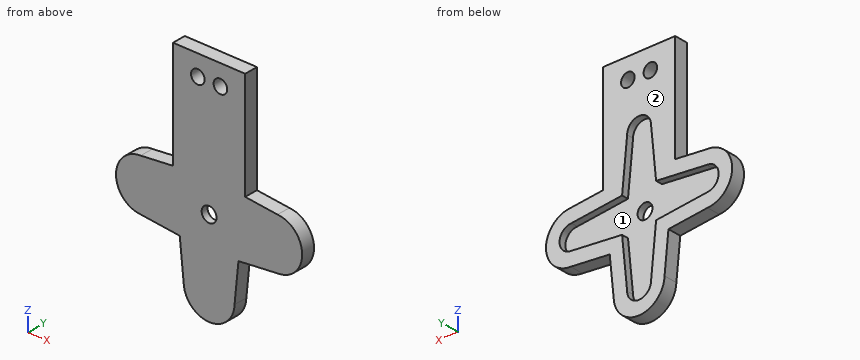
```python
from build123d import *
from build123d.topology import SkipClean

# Parameters (mm, degrees)
SKETCH1_R               = 21
BOSS_EXTRUDE1_DEPTH     = 1.5
SKETCH2_R               = 2.65
CUT_EXTRUDE1_DEPTH      = 1.5
SKETCH5_W               = 16
SKETCH5_H               = 30
BOSS_EXTRUDE2_DEPTH     = 1.5
CIRPATTERN1_DEPTH       = 1.5
CUT_EXTRUDE4_REACH      = 38.65
SKETCH4_R               = 1.65
CUT_EXTRUDE5_REACH      = 38.742
SKETCH6_R               = 1.5
CUT_EXTRUDE6_DEPTH      = 37.650375169
CUT_EXTRUDE6_DEPTH_BACK = 37.650375169


# Read off the part's stored shape, not the designer's step: CirPattern1
with BuildPart() as part:
    # Sketch1 → Boss-Extrude1 (new, symmetric)
    with BuildSketch(Plane(origin=(0, 0, 0), x_dir=(1, 0, 0), z_dir=(0, 1, 0))):
        with Locations(Location((0, 0, 0), (0, 0, 270))):
            Circle(SKETCH1_R)
    extrude(amount=BOSS_EXTRUDE1_DEPTH, both=True)

    # Sketch2 → Cut-Extrude1 (cut)
    with BuildSketch(Plane(origin=(0, 1.5, 0), x_dir=(1, 0, 0), z_dir=(0, 1, 0))):
        with Locations((0, -15)):
            Circle(SKETCH2_R)
        with BuildLine():
            ThreePointArc((-2.65, -15), (0, -12.35), (2.65, -15))
            Line((2.65, -15), (4.067821782, -0.821782178))
            ThreePointArc((4.067821782, -0.821782178), (0, -4.15), (-4.067821782, -0.821782178))
            Line((-4.067821782, -0.821782178), (-2.65, -15))
        make_face()
        with BuildLine():
            ThreePointArc((-4.067821782, -0.821782178), (0, -4.15), (4.067821782, -0.821782178))
            Line((4.067821782, -0.821782178), (4.15, 0))
            ThreePointArc((4.15, 0), (0, 4.15), (-4.15, 0))
            Line((-4.15, 0), (-4.067821782, -0.821782178))
        make_face()
    cut_extrude1 = extrude(amount=-CUT_EXTRUDE1_DEPTH, mode=Mode.SUBTRACT)

    # Sketch5 → Boss-Extrude2 (add, symmetric)
    with BuildSketch(Plane(origin=(0, 0, 0), x_dir=(1, 0, 0), z_dir=(0, 1, 0))):
        with Locations((0, -15)):
            Rectangle(SKETCH5_W, SKETCH5_H)
    extrude(amount=BOSS_EXTRUDE2_DEPTH, both=True)

    # Mirror1: Cut-Extrude1 across plane
    with SkipClean():  # the faces are left unmerged after this step: merging them gives an invalid solid
        add(cut_extrude1.mirror(Plane.XY), mode=Mode.SUBTRACT)

    # CirPattern1 outline → CirPattern1 (cut)
    with BuildSketch(Plane(origin=(0, 0, 0), x_dir=(1, 0, 0), z_dir=(0, 1, 0))):
        with BuildLine():
            Line((3.772727273, -3.772727273), (15, -2.65))
            ThreePointArc((15, -2.65), (17.65, 0), (15, 2.65))
            Line((15, 2.65), (3.772727273, 3.772727273))
            Line((3.772727273, 3.772727273), (4.067821782, 0.821782178))
            ThreePointArc((4.067821782, 0.821782178), (0, -4.15), (-4.067821782, 0.821782178))
            Line((-4.067821782, 0.821782178), (-3.772727273, 3.772727273))
            Line((-3.772727273, 3.772727273), (-15, 2.65))
            ThreePointArc((-15, 2.65), (-17.65, 0), (-15, -2.65))
            Line((-15, -2.65), (-3.772727273, -3.772727273))
            Line((-3.772727273, -3.772727273), (-2.65, -15))
            ThreePointArc((-2.65, -15), (0, -17.65), (2.65, -15))
            Line((2.65, -15), (3.772727273, -3.772727273))
        make_face()
    extrude(amount=CIRPATTERN1_DEPTH, mode=Mode.SUBTRACT)

    # Sketch4 → Cut-Extrude4 (cut, up to next)
    with BuildSketch(Plane(origin=(0, 0, 0), x_dir=(1, 0, 0), z_dir=(0, 1, 0)), mode=Mode.PRIVATE) as cut_extrude4_sk1:
        with Locations(Location((0, 0, 0), (0, 0, 270))):
            Circle(SKETCH4_R)
    cut_extrude4_tool1 = extrude(cut_extrude4_sk1.sketch, amount=-CUT_EXTRUDE4_REACH, mode=Mode.PRIVATE) & part.part
    add(cut_extrude4_tool1.solids().sort_by_distance((0, 0, 0))[0], mode=Mode.SUBTRACT)

    # Sketch6 → Cut-Extrude5 (cut, up to next)
    with BuildSketch(Plane(origin=(0, 1.5, 0), x_dir=(1, 0, 0), z_dir=(0, 1, 0)), mode=Mode.PRIVATE) as cut_extrude5_sk1:
        with Locations(Location((2.5, -25.5, 0), (0, 0, 270))):
            Circle(SKETCH6_R)
    cut_extrude5_tool1 = extrude(cut_extrude5_sk1.sketch, amount=-CUT_EXTRUDE5_REACH, mode=Mode.PRIVATE) & part.part
    # Sketch6 → Cut-Extrude5 (cut, up to next)
    with BuildSketch(Plane(origin=(0, 1.5, 0), x_dir=(1, 0, 0), z_dir=(0, 1, 0)), mode=Mode.PRIVATE) as cut_extrude5_sk2:
        with Locations(Location((-2.5, -25.5, 0), (0, 0, 270))):
            Circle(SKETCH6_R)
    cut_extrude5_tool2 = extrude(cut_extrude5_sk2.sketch, amount=-CUT_EXTRUDE5_REACH, mode=Mode.PRIVATE) & part.part
    add(cut_extrude5_tool1.solids().sort_by_distance((2.5, 1.5, 25.5))[0], mode=Mode.SUBTRACT)
    add(cut_extrude5_tool2.solids().sort_by_distance((-2.5, 1.5, 25.5))[0], mode=Mode.SUBTRACT)

    # Sketch7 → Cut-Extrude6 (cut, two sides: drawn at the far end of the back side and taken through both)
    with BuildSketch(Plane(origin=(0, 0, 0), x_dir=(1, 0, 0), z_dir=(0, 1, 0)).offset(-CUT_EXTRUDE6_DEPTH_BACK)):
        with BuildLine():
            ThreePointArc((8, -19.416487839), (0, 21), (-8, -19.416487839))
            Line((-8, -19.416487839), (-8, -6.364962686))
            Line((-8, -6.364962686), (-15.177522436, -5.647210443))
            ThreePointArc((-15.177522436, -5.647210443), (-20.65, 0), (-15.177522436, 5.647210443))
            Line((-15.177522436, 5.647210443), (-6.513602442, 6.513602442))
            Line((-6.513602442, 6.513602442), (-5.647210443, 15.177522436))
            ThreePointArc((-5.647210443, 15.177522436), (0, 20.65), (5.647210443, 15.177522436))
            Line((5.647210443, 15.177522436), (6.513602442, 6.513602442))
            Line((6.513602442, 6.513602442), (15.177522436, 5.647210443))
            ThreePointArc((15.177522436, 5.647210443), (20.65, 0), (15.177522436, -5.647210443))
            Line((15.177522436, -5.647210443), (8, -6.364962686))
            Line((8, -6.364962686), (8, -19.416487839))
        make_face()
    extrude(amount=CUT_EXTRUDE6_DEPTH + CUT_EXTRUDE6_DEPTH_BACK, mode=Mode.SUBTRACT)


solid = part.part
```
Design review of the part built by this model. Coordinates are the model's own, in mm. Face numbers are marked on the shaded views. Give positions to 0.01 mm unless a question says otherwise; leave off trailing zeros. Loops run counter-clockwise (first coordinate to the right, second up) from the corner with the lowest first, then second, coordinate; pieces in that order, holes last. Notation, with made-up numbers: (33, 62) -> (86, 62) arc R27 ccw to (86, 85) -> close; hole circle Ø4 at (-3.5, 55). An arc over 180 degrees is marked (long way). Write each question's results on one line, items separated by ' | '.
Q1. Wall thickness on L1, parallel to X at y = -0.7, z = 25.5; L2, parallel to Z at x = 2, y = 0.35; L3, parallel to X at y = -1.05, z = 0: over which ranges is each line inside the solid? List them lowest first.
Reply:
L1: x = -8 to -4, -1 to 1, 4 to 8 | L2: z = -20.28 to -16.74, 16.74 to 24.09, 26.91 to 30 | L3: x = -20.65 to -1.65, 1.65 to 20.65
Q2. Take a section at B-B, the plane z = 25.5. Write out the cut boundary in (x, y).
Reply:
outline: (-8, -1.5) -> (-4, -1.5) -> (-4, 1.5) -> (-8, 1.5) -> close; (-1, -1.5) -> (1, -1.5) -> (1, 1.5) -> (-1, 1.5) -> close; (4, -1.5) -> (8, -1.5) -> (8, 1.5) -> (4, 1.5) -> close
Q3. For pin 1 Ø0.9 at (y, z) = (0.5, 12.5) entering from +X; pin 2 Ø1.8 at (x, z) = (-2.5, 25.5) entering from -Y, all flat-tipped, find the tip position at first contact; note any pin that passes through.
Reply:
pin 1: stops at x = 8 | pin 2: passes through
Q4. The part is to be moulded in two halves that separate along Z. For the marked faces 1 and 2, say which applies: +Z half, -Z half, draft (parallel to the pull), parting line (faces both ways), or undercut.
Reply:
face 1: undercut | face 2: draft
Q5. Take a section at D-D, the plane z = 10. Write out the cut boundary in (x, y).
Reply:
outline: (-8, -1.5) -> (8, -1.5) -> (8, 1.5) -> (3.15, 1.5) -> (3.15, 0) -> (-3.15, 0) -> (-3.15, 1.5) -> (-8, 1.5) -> close
Q6. Take a section at A-A, the plane x = 0. Write out the cut boundary in (y, z).
Reply:
outline: (-1.5, -20.65) -> (1.5, -20.65) -> (1.5, -17.65) -> (0, -17.65) -> (0, -1.65) -> (-1.5, -1.65) -> close; (-1.5, 1.65) -> (0, 1.65) -> (0, 17.65) -> (1.5, 17.65) -> (1.5, 30) -> (-1.5, 30) -> close
